Geometry check sheet. Reference: the model listing, model coordinates, mm. Give positions to 0.01 mm unless a question says otherwise; leave off trailing zeros. Order: outer loops, then holes, each group sorted by start corner. A loop starts at its lowest first (then second) coordinate and runs counter-clockwise, first axis right, second up.
from build123d import *

# Parameters (mm, degrees)
SKETCH1_W                   = 876.3
SKETCH1_H                   = 571.5
BOSS_EXTRUDE1_DEPTH         = 2.54
F_1_4_0_25_DIAMETER_HOLE1_D = 6.35
LPATTERN1_COUNT             = 6
LPATTERN1_PITCH             = 114.3


with BuildPart() as part:
    # Sketch1 → Boss-Extrude1 (new body)
    with BuildSketch(Plane(origin=(0, 0, 0), x_dir=(1, 0, 0), z_dir=(0, 1, 0))):
        Polygon((-472.44, -320.04), (472.44, -320.04), (472.44, 320.04), (-472.44, 320.04), (-476.25, 320.04), (-476.25, -320.04), align=None)
        Rectangle(SKETCH1_W, SKETCH1_H, mode=Mode.SUBTRACT)
    extrude(amount=BOSS_EXTRUDE1_DEPTH)

    # 1/4 (0.25) Diameter Hole1 (through all)
    with Locations(Plane(origin=(-468.63, 2.54, -285.75), x_dir=(0, 0, 1), z_dir=(0, 1, 0))):
        with Locations((0, 0)):
            f_1_4_0_25_diameter_hole1 = Hole(F_1_4_0_25_DIAMETER_HOLE1_D / 2)

    # LPattern1: 1/4 (0.25) Diameter Hole1 ×6
    with Locations(*[(0, 0, i * LPATTERN1_PITCH) for i in range(1, LPATTERN1_COUNT)]):
        add(f_1_4_0_25_diameter_hole1, mode=Mode.SUBTRACT)


solid = part.part
Item 1: Sectioned sample at A-A (z = 135.5). Enter the section's corners in (x, y), and give its area (3 significant figures).
Reported:
outline: (-476.25, 0) - (-438.15, 0) - (-438.15, 2.54) - (-476.25, 2.54) - close; (438.15, 0) - (472.44, 0) - (472.44, 2.54) - (438.15, 2.54) - close
area: 184 mm2
Item 2: Sectioned sample at B-B (x = 164). Enter the section's corners in (y, z).
Reported:
outline: (0, -320.04) - (2.54, -320.04) - (2.54, -285.75) - (0, -285.75) - close; (0, 285.75) - (2.54, 285.75) - (2.54, 320.04) - (0, 320.04) - close
Item 3: Scan lines: L1, parallel to X at y = 1.2, z = 171.45 (3 decimals); L2, parallel to Z at x = -34, y = 0.85; L3, parallel to X at y = 2.05, z = -40. Record each from-to range of solid material in increasing order.
Reported:
L1: x = -476.25 to -471.805, -465.455 to -438.15, 438.15 to 472.44
L2: z = -320.04 to -285.75, 285.75 to 320.04
L3: x = -476.25 to -438.15, 438.15 to 472.44
Item 4: Sectioned sample at C-C (y = 2.15). Enter the section's corners in (x, z) (3 decimals).
Reported:
outline: (-476.25, -320.04) - (472.44, -320.04) - (472.44, 320.04) - (-476.25, 320.04) - close; hole circle Ø6.35 at (-468.63, -285.75); hole circle Ø6.35 at (-468.63, -171.45); hole circle Ø6.35 at (-468.63, -57.15); hole circle Ø6.35 at (-468.63, 57.15); hole circle Ø6.35 at (-468.63, 171.45); hole circle Ø6.35 at (-468.63, 285.75); hole (-438.15, -285.75) - (438.15, -285.75) - (438.15, 285.75) - (-438.15, 285.75) - close
Item 5: Gauge pin test, flat ends, axial feed: pin 1 (7.5 mm diameter, centred on x = -468.63, z = -171.45, fed in from +Y); pin 2 (5 mm diameter, centred on x = -468.63, z = 57.15, fed in from -Y). Record the tip position at first contact, or that the pin passes through.
Reported:
pin 1: stops at y = 2.54
pin 2: passes through
